Could you check a few things on this drawing? It's one solid part, dimensions in mm from its lowest x, y, z. A direction names the side the tool comes from. Round coordinates to 2 decimals unless told otherwise and drop trailing zeros. Loops run counter-clockwise (first coordinate to the right, second up) from the corner with the lowest first, then second, coordinate; pieces in that order, holes last. Notation, with made-up numbers: M 71,71.25 L 119,71.25 A8 cw 119,83.25 Z; hole C -37.75,51.5 d8. An arc over 180 degrees is marked long. Write item = value, one per line. Start each with the question number.
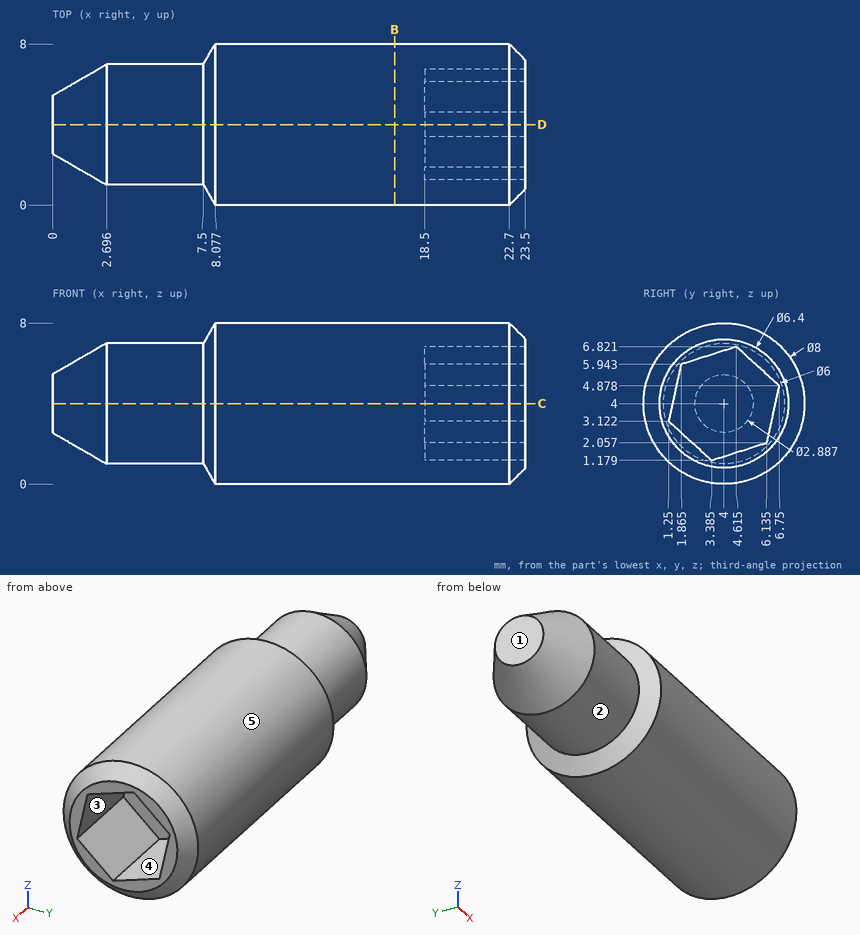
Item 1: Please list where these lines run through material, in increasing order: line 1 (X direction, y = 5, z = 3.75); line 2 (Z direction, x = 20.75, y = 6) (1 decimal); line 3 (Y direction, x = 19, z = 4). Write a range as [from, to].
Item 2: For the marked faces 4 and 5, which set-ups out of +Z, -Z, +X, -X, +Y, -Y let a thin tool reach every point of the face, with its end or its side?
Item 3: I want a section at D-D, the plane y = 4. List the corners of the cut face in (x, z) for me (1 decimal).
Item 4: I want a section at C-C, the plane z = 4. List the corners of the cut face in (x, y) for me, then the cut area to 3 significant figures.
Item 5: We'd pull the mould along Y, two halves only. Please class the marked faces 1, 2 and 3: released by +Y, released by -Y, zero draft, split by the parting line, or undercut.
Item 6: I want a section at B-B, the plane x = 17. List the corners of the cut face in (y, z) for me.
Item 7: Will these pins go through, and if not, where does the flat tip stop? pin 1 Ø1.5 at (y, z) = (2, 7) entering from +X; pin 2 Ø3 at (x, z) = (19.5, 1) entering from -Y; pin 3 Ø1 at (x, z) = (13.5, 1) entering from -Y; pin 4 Ø2 at (x, y) = (19, 6.5) entering from +Z.
Worked out:
q1.line_1 = [0, 18.5]
q1.line_2 = [0.5, 2], [5.6, 7.5]
q1.line_3 = [0, 1.44], [6.56, 8]
q2.face_4 = +X
q2.face_5 = +X, -X
q3.outline = M 0,2.6 L 2.7,1 L 7.5,1 L 8.1,0 L 22.7,0 L 23.5,0.8 L 23.5,1.4 L 18.5,1.4 L 18.5,6.6 L 23.5,6.6 L 23.5,7.2 L 22.7,8 L 8.1,8 L 7.5,7 L 2.7,7 L 0,5.4 Z
q4.outline = M 0,2.56 L 2.7,1 L 7.5,1 L 8.08,0 L 22.7,0 L 23.5,0.8 L 23.5,1.44 L 18.5,1.44 L 18.5,6.56 L 23.5,6.56 L 23.5,7.2 L 22.7,8 L 8.08,8 L 7.5,7 L 2.7,7 L 0,5.44 Z
q4.area = 142 mm2
q5.face_1 = zero draft
q5.face_2 = split by the parting line
q5.face_3 = undercut
q6.outline = C 4,4 d8
q7.pin_1 = 23.5
q7.pin_2 = 0.29
q7.pin_3 = 0.88
q7.pin_4 = 7.71
